```python
from build123d import *

# Parameters (mm, degrees)
SKIZZE1_W                       = 40
SKIZZE1_H                       = 110
AUFSATZ_LINEAR_AUSTRAGEN1_DEPTH = 10
SKIZZE2_W                       = 40
SKIZZE2_H                       = 43
SCHNITT_LINEAR_AUSTRAGEN1_DEPTH = 3
SKIZZE3_R                       = 2.75
SCHNITT_LINEAR_AUSTRAGEN2_DEPTH = 11
SKIZZE5_R                       = 11
SCHNITT_LINEAR_AUSTRAGEN4_DEPTH = 8
SKIZZE6_R                       = 10
SCHNITT_LINEAR_AUSTRAGEN5_DEPTH = 8
FASE1_SIZE                      = 1
SKIZZE10_W                      = 40
SKIZZE10_H                      = 10
AUFSATZ_LINEAR_AUSTRAGEN2_DEPTH = 9.7
SKIZZE11_R                      = 3
SCHNITT_LINEAR_AUSTRAGEN6_DEPTH = 21
SKIZZE12_R                      = 4.5
SCHNITT_LINEAR_AUSTRAGEN7_DEPTH = 13
SKIZZE13_R                      = 11.25
SCHNITT_LINEAR_AUSTRAGEN8_DEPTH = 3


with BuildPart() as part:
    # Skizze1 → Aufsatz-Linear austragen1 (new body)
    with BuildSketch(Plane.XY):
        with Locations((20, 55)):
            Rectangle(SKIZZE1_W, SKIZZE1_H)
    extrude(amount=AUFSATZ_LINEAR_AUSTRAGEN1_DEPTH)

    # Skizze2 → Schnitt-Linear austragen1 (cut)
    with BuildSketch(Plane(origin=(0, 0, 0), x_dir=(-1, 0, 0), z_dir=(0, 0, -1))):
        with Locations((-20, 31.5)):
            Rectangle(SKIZZE2_W, SKIZZE2_H)
    extrude(amount=-SCHNITT_LINEAR_AUSTRAGEN1_DEPTH, mode=Mode.SUBTRACT)

    # Skizze3 → Schnitt-Linear austragen2 (cut)
    with BuildSketch(Plane(origin=(0, 0, 3), x_dir=(-1, 0, 0), z_dir=(0, 0, -1))):
        with Locations((-20, 31.5)):
            Circle(SKIZZE3_R)
    extrude(amount=-SCHNITT_LINEAR_AUSTRAGEN2_DEPTH, mode=Mode.SUBTRACT)

    # Skizze5 → Schnitt-Linear austragen4 (cut)
    with BuildSketch(Plane.XY.offset(10)):
        with Locations((20.290455997, 96.4)):
            Circle(SKIZZE5_R)
    extrude(amount=-SCHNITT_LINEAR_AUSTRAGEN4_DEPTH, mode=Mode.SUBTRACT)

    # Skizze6 → Schnitt-Linear austragen5 (cut)
    with BuildSketch(Plane.XY.offset(2)):
        with Locations((20.290455997, 96.4)):
            Circle(SKIZZE6_R)
    extrude(amount=-SCHNITT_LINEAR_AUSTRAGEN5_DEPTH, mode=Mode.SUBTRACT)

    # Fase1
    fase1_edges = [part.edges().sort_by_distance(p)[0] for p in [
        (22.75, 31.5, 10),
        (9.290455997, 96.4, 10),
    ]]
    chamfer(fase1_edges, length=FASE1_SIZE)

    # Skizze10 → Aufsatz-Linear austragen2 (add)
    with BuildSketch(Plane.XY.offset(10)):
        with Locations((20, 5)):
            Rectangle(SKIZZE10_W, SKIZZE10_H)
    extrude(amount=AUFSATZ_LINEAR_AUSTRAGEN2_DEPTH)

    # Skizze11 → Schnitt-Linear austragen6 (cut)
    with BuildSketch(Plane(origin=(0, 0, 0), x_dir=(-1, 0, 0), z_dir=(0, 0, -1))):
        with Locations((-32.5, 5)):
            Circle(SKIZZE11_R)
        with Locations((-7.5, 5)):
            Circle(SKIZZE11_R)
    extrude(amount=-SCHNITT_LINEAR_AUSTRAGEN6_DEPTH, mode=Mode.SUBTRACT)

    # Skizze12 → Schnitt-Linear austragen7 (cut)
    with BuildSketch(Plane(origin=(0, 0, 0), x_dir=(-1, 0, 0), z_dir=(0, 0, -1))):
        with Locations((-32.5, 5)):
            Circle(SKIZZE12_R)
        with Locations((-7.5, 5)):
            Circle(SKIZZE12_R)
    extrude(amount=-SCHNITT_LINEAR_AUSTRAGEN7_DEPTH, mode=Mode.SUBTRACT)

    # Skizze13 → Schnitt-Linear austragen8 (cut)
    with BuildSketch(Plane(origin=(0, 0, 3), x_dir=(-1, 0, 0), z_dir=(0, 0, -1))):
        with Locations((-20, 31.5)):
            Circle(SKIZZE13_R)
    extrude(amount=-SCHNITT_LINEAR_AUSTRAGEN8_DEPTH, mode=Mode.SUBTRACT)


solid = part.part
```
For this review, take the finished solid that the model builds, in its own axes (mm). A direction names the side the tool comes from. Give positions to 0.01 mm unless a question says otherwise; leave off trailing zeros. Write each loop counter-clockwise with the first axis right and the second up, starting at its lowest first coordinate (ties: lowest second). Pieces come first, ordered by that corner, then holes. Notation, with made-up numbers: M 74.25,62 L 99.25,62 A10 cw 99.25,68 Z; hole C -23.75,59.25 d1. An arc over 180 degrees is marked long. Answer as a JSON object with one key per item and string values. Group by question number.
Item 1: Consider section B-B on z = 17.5. Write out the cut boundary in (x, y), plus the area to 3 significant figures.
Item 2: Consider section D-D on x = 20. Count the separate pieces of the cut face and the enclosed holes in it, plus the area to 3 significant figures.
Item 3: For probe 1 along Y at (x, z) = (20, 7.7); probe 2 along Y at (x, z) = (20, 4.35); probe 3 along Y at (x, z) = (7.5, 10.25), list the stretches that pass through material, from the lowest coordinate up. Write a range as [from, to].
Item 4: Draft analysis for pull direction Y (two halves, no side actions). For faces 5 (the flat face through (20, 10, 15)), 6 (the cylindrical face through (28.34, 3.28, 6.41)), 7 (the flat face through (20, 5, 0)), state which applies: +Y half, -Y half, draft (parallel to the pull), parting line (faces both ways), or undercut.
Item 5: For pin 1 Ø12 at (x, y) = (27.5, 34.5) entering from +Z; pin 2 Ø20 at (x, y) = (20, 25.5) entering from -Z; pin 3 Ø3 at (y, z) = (39.5, 6) entering from -X; pin 4 Ø7 at (x, y) = (32.5, 5) entering from -Z, all flat-tipped, find the tip position at first contact; note any pin that passes through.
Item 6: Consider section A-A on y = 96.4. Write out the cut boundary in (x, z), plus the area to 3 significant figures.
Item 7: Tool access review of faces 1 (the flat face through (20, 61, 10)), 2 (the flat face through (18, 29, 6)), 3 (the flat face through (25, 87, 2)), 4 (the flat face through (11, 22, 3)): name each direction out of +Z, -Z, +X, -X, +Y, -Y from which nothing blocks a thin tool from reaching the whole face with its end or side.
Item 8: Consider section C-C on y = 31.5. Write out the cut boundary in (x, z).
Check result:
{
 "1": {"outline": "M 0,0 L 40,0 L 40,10 L 0,10 Z; hole C 7.5,5 d6; hole C 32.5,5 d6", "area": "343 mm^2"},
 "2": {"separate pieces": "3", "enclosed holes": "0", "area": "761 mm^2"},
 "3": {"probe 1": "y = [0, 28.75], [34.25, 85.4], [107.4, 110]", "probe 2": "y = [0, 20.25], [42.75, 85.4], [107.4, 110]", "probe 3": "y = [0, 0.5], [9.5, 10]"},
 "4": {"face 5": "+Y half", "face 6": "undercut", "face 7": "draft"},
 "5": {"pin 1": "stops at z = 10", "pin 2": "stops at z = 3", "pin 3": "stops at x = 0", "pin 4": "stops at z = 13"},
 "6": {"outline": "M 0,0 L 10.29,0 L 10.29,2 L 9.29,2 L 9.29,9 L 8.29,10 L 0,10 Z; M 30.29,0 L 40,0 L 40,10 L 32.29,10 L 31.29,9 L 31.29,2 L 30.29,2 Z", "area": "183 mm^2"},
 "7": {"face 1": "+Z, +X, -X, +Y", "face 2": "-Z", "face 3": "+Z", "face 4": "-Z, +X, -X"},
 "8": {"outline": "M 0,3 L 8.75,3 L 8.75,6 L 17.25,6 L 17.25,9 L 16.25,10 L 0,10 Z; M 22.75,6 L 31.25,6 L 31.25,3 L 40,3 L 40,10 L 23.75,10 L 22.75,9 Z"}
}
